Job drawing, mm, ordinate dimensions from the low corner. One solid piece. A direction names the side the tool comes from. Round coordinates to 2 decimals unless told otherwise and drop trailing zeros. Write each loop counter-clockwise with the first axis right and the second up, starting at its lowest first coordinate (ties: lowest second). Pieces come first, ordered by that corner, then holes.
1) Saw through at B-B (z = 93.5). Write the cut outline in (x, y) (1 decimal), plus the area to 3 significant figures.
2) Flat gauge pins, fed straight in: pin 1 (6 mm diameter, centred on x = 135.5, y = 2.5, fed in from +Z); pin 2 (22 mm diameter, centred on x = 117, z = 69, fed in from +Y); pin 3 (5 mm diameter, centred on y = 20.5, z = 43.5, fed in from +X); pin 4 (8 mm diameter, centred on y = 15.5, z = 155.5, fed in from -X). Where does each tip first touch, or does it go through?
3) Saw through at A-A (x = 97.5). Write the cut outline in (y, z), plus the area to 3 significant figures.
4) Saw through at D-D (y = 12). Write the cut outline in (x, z) (1 decimal).
5) Saw through at C-C (y = 2.25). Write the cut outline in (x, z), plus the area to 3 significant figures.
6) Which spindle directions (+Z, -Z, +X, -X, +Y, -Y) get a long thin tool onto all of the face, cutting with end or side? Do the marked faces 1 and 2. Say none if no direction does.
7) Wall check: probe 1 along Y at (x, z) = (119, 76); probe 2 along Z at (x, y) = (106, 21.25) (1 decimal); probe 3 along X at (y, z) = (20, 125.5). Give the ranges that are in metal, low to high.
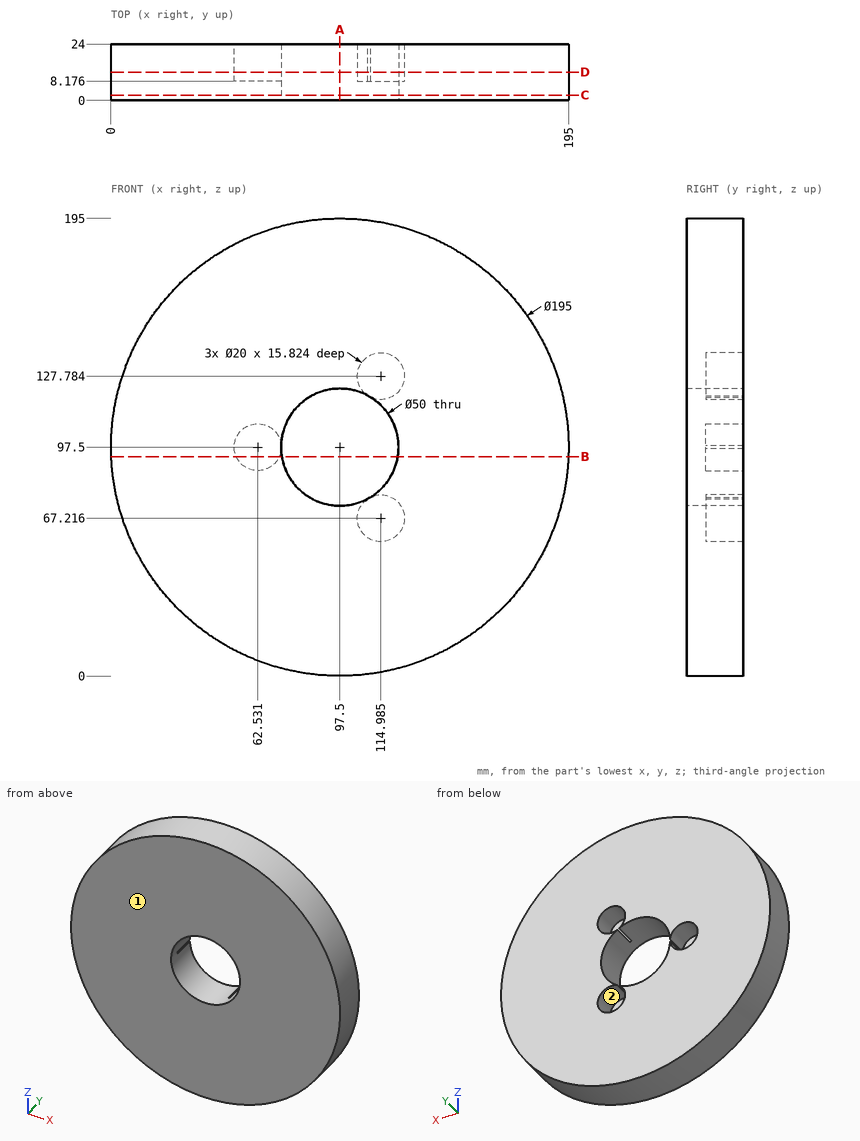
Evaluation:
1. outline: (0.1, 0) - (72.8, 0) - (72.8, 24) - (71.7, 24) - (71.7, 8.2) - (53.4, 8.2) - (53.4, 24) - (0.1, 24) - close; (122.2, 0) - (194.9, 0) - (194.9, 24) - (122.2, 24) - close
1. area: 3,200 mm2
2. pin 1: stops at z = 188.5
2. pin 2: stops at y = 24
2. pin 3: stops at x = 180.29
2. pin 4: stops at x = 16.32
3. outline: (0, 0) - (24, 0) - (24, 72.5) - (0, 72.5) - close; (0, 122.5) - (24, 122.5) - (24, 195) - (0, 195) - close
3. area: 3,480 mm2
4. outline: circle Ø195 at (97.5, 97.5); hole (72.5, 96.8) arc R25 ccw to (109.4, 75.5) arc R10 ccw (long way) to (110.6, 76.2) arc R25 ccw to (110.6, 118.8) arc R10 ccw (long way) to (109.4, 119.5) arc R25 ccw to (72.5, 98.2) arc R10 ccw (long way) to start
5. outline: circle Ø195 at (97.5, 97.5); hole circle Ø50 at (97.5, 97.5)
5. area: 27,900 mm2
6. face 1: +Z, -Z, +X, -X, -Y
6. face 2: +Y
7. probe 1: y = 0 to 8.18
7. probe 2: z = 0.4 to 62.8, 71.6 to 74, 121 to 123.4, 132.2 to 194.6
7. probe 3: x = 4.11 to 105.25, 124.72 to 190.89
